from build123d import *

# Parameters (mm, degrees)
SKETCH8_R            = 1.55
BASE_FLANGE2_DEPTH   = 2.42
M3_CLEARANCE_HOLE3_D = 3.4


# Sheet-metal steps are written as plain solids
with BuildPart() as part:
    # Sketch8 → Base-Flange2 (new body)
    with BuildSketch(Plane(origin=(0, 0, 0), x_dir=(1, 0, 0), z_dir=(0, 1, 0))):
        with BuildLine():
            Line((27.763932023, 19.472135955), (-2.236067977, 4.472135955))
            ThreePointArc((-2.236067977, 4.472135955), (-5, 0), (-2.236067977, -4.472135955))
            Line((-2.236067977, -4.472135955), (27.763932023, -19.472135955))
            ThreePointArc((27.763932023, -19.472135955), (34.472135955, -17.236067977), (32.236067977, -10.527864045))
            Line((32.236067977, -10.527864045), (14.758048651, -1.788854382))
            ThreePointArc((14.758048651, -1.788854382), (13.652475842, 0), (14.758048651, 1.788854382))
            Line((14.758048651, 1.788854382), (32.236067977, 10.527864045))
            ThreePointArc((32.236067977, 10.527864045), (34.472135955, 17.236067977), (27.763932023, 19.472135955))
        make_face()
        with Locations(Location((0, 0, 0), (0, 0, 270))):
            Circle(SKETCH8_R, mode=Mode.SUBTRACT)
    extrude(amount=-BASE_FLANGE2_DEPTH)

    # M3 Clearance Hole3 (through all)
    with Locations(Plane(origin=(0, 0, 0), x_dir=(1, 0, 0), z_dir=(0, 1, 0))):
        with Locations((30, 15), (30, -15)):
            Hole(M3_CLEARANCE_HOLE3_D / 2)


solid = part.part
Model file for the job. Use its own axes, mm. A direction names the side the tool comes from. Round coordinates to 2 decimals unless told otherwise and drop trailing zeros. Order: outer loops, then holes, each group sorted by start corner. A loop starts at its lowest first (then second) coordinate and runs counter-clockwise, first axis right, second up.
(1) Pull direction Z, two halves, no side cores. Call faces 1 (the face through (0.466, -1.193, 1.478)), 2 (the face through (19, -2.42, -5)), 3 (the face through (-5, -1, 0)): released by +Z, released by -Z, zero draft, split by the parting line, or undercut.
(2) 3-axis set-ups, long thin cutter, end or side, ignore diameter. For faces 4 (the face through (23.375, -1.193, -6.097)), 5 (the face through (28.43, -1.23, 15.65)): which of +Z, -Z, +X, -X, +Y, -Y reach the whole face in a straight line?
(3) Band-saw the part on C-C (x = 30). List the corners of the cut face in (y, z).
(4) Band-saw the part on B-B (y = -1.7). List the corners of the cut face in (x, z).
(5) Drill centre lines: line 1 (Z direction, x = 30, y = -1.1); line 2 (Z direction, x = 22.5, y = -1.85); line 3 (Z direction, x = 22, y = -0.4). Where is each one in solid material? Low to high.
(6) Band-saw the part on D-D (x = 22.5). List the corners of the cut face in (y, z).
(7) Band-saw the part on A-A (z = 0). List the corners of the cut face in (x, y), then the cut area to 3 significant figures.
(8) Pin check, flat tip, straight feed: pin 1 (4 mm diameter, centred on x = 0, z = 0, fed in from -Y). Stop position of the tip, or through.
Verdict:
1. face 1: undercut
1. face 2: zero draft
1. face 3: split by the parting line
2. face 4: +X, +Y, -Y
2. face 5: +Y, -Y
3. outline: (-2.42, -20) - (0, -20) - (0, -16.7) - (-2.42, -16.7) - close; (-2.42, -13.3) - (0, -13.3) - (0, -9.41) - (-2.42, -9.41) - close; (-2.42, 9.41) - (0, 9.41) - (0, 13.3) - (-2.42, 13.3) - close; (-2.42, 16.7) - (0, 16.7) - (0, 20) - (-2.42, 20) - close
4. outline: (-2.24, -4.47) - (27.76, -19.47) arc R5 ccw to (32.24, -10.53) - (14.76, -1.79) arc R2 cw to (14.76, 1.79) - (32.24, 10.53) arc R5 ccw to (27.76, 19.47) - (-2.24, 4.47) arc R5 ccw to start; hole circle Ø3.1 at (0, 0); hole circle Ø3.4 at (30, -15); hole circle Ø3.4 at (30, 15)
5. line 1: z = -20 to -16.7, -13.3 to -9.41, 9.41 to 13.3, 16.7 to 20
5. line 2: z = -16.84 to -5.66, 5.66 to 16.84
5. line 3: z = -16.59 to -5.41, 5.41 to 16.59
6. outline: (-2.42, -16.84) - (0, -16.84) - (0, -5.66) - (-2.42, -5.66) - close; (-2.42, 5.66) - (0, 5.66) - (0, 16.84) - (-2.42, 16.84) - close
7. outline: (-5, -2.42) - (-1.55, -2.42) - (-1.55, 0) - (-5, 0) - close; (1.55, -2.42) - (13.65, -2.42) - (13.65, 0) - (1.55, 0) - close
7. area: 37.6 mm2
8. pin 1: stops at y = -2.42
